```python
from build123d import *

# Parameters (mm, degrees)
SKETCH1_W           = 50
SKETCH1_H           = 40
BOSS_EXTRUDE1_DEPTH = 6
CUT_EXTRUDE3_DEPTH  = 4
SKETCH7_R           = 2
CUT_EXTRUDE4_DEPTH  = 6


with BuildPart() as part:
    # Sketch1 → Boss-Extrude1 (new body)
    with BuildSketch(Plane.XY):
        Rectangle(SKETCH1_W, SKETCH1_H)
    extrude(amount=BOSS_EXTRUDE1_DEPTH)

    # Sketch6 → Cut-Extrude3 (cut)
    with BuildSketch(Plane(origin=(0, 0, 0), x_dir=(-1, 0, 0), z_dir=(0, 0, -1))):
        with BuildLine():
            Line((-16.5, 15), (-16.5, -6))
            ThreePointArc((-16.5, -6), (-20, -9.5), (-23.5, -6))
            Line((-23.5, -6), (-23.5, 15))
            ThreePointArc((-23.5, 15), (-20, 18.5), (-16.5, 15))
        make_face()
        with BuildLine():
            Line((23.5, 15), (23.5, -6))
            ThreePointArc((23.5, -6), (20, -9.5), (16.5, -6))
            Line((16.5, -6), (16.5, 15))
            ThreePointArc((16.5, 15), (20, 18.5), (23.5, 15))
        make_face()
    extrude(amount=-CUT_EXTRUDE3_DEPTH, mode=Mode.SUBTRACT)

    # Sketch7 → Cut-Extrude4 (cut)
    with BuildSketch(Plane(origin=(0, 0, 0), x_dir=(-1, 0, 0), z_dir=(0, 0, -1))):
        with Locations((-20, -16.5)):
            Circle(SKETCH7_R)
        with Locations((20, -16.5)):
            Circle(SKETCH7_R)
        with BuildLine():
            Line((-22, 15), (-22, -6))
            ThreePointArc((-22, -6), (-20, -8), (-18, -6))
            Line((-18, -6), (-18, 15))
            ThreePointArc((-18, 15), (-20, 17), (-22, 15))
        make_face()
        with BuildLine():
            Line((18, 15), (18, -6))
            ThreePointArc((18, -6), (20, -8), (22, -6))
            Line((22, -6), (22, 15))
            ThreePointArc((22, 15), (20, 17), (18, 15))
        make_face()
    extrude(amount=-CUT_EXTRUDE4_DEPTH, mode=Mode.SUBTRACT)


solid = part.part
```
Part model, mm, in its own coordinate system. A direction names the side the tool comes from. Give positions to 0.01 mm unless a question says otherwise; leave off trailing zeros. Order: outer loops, then holes, each group sorted by start corner. A loop starts at its lowest first (then second) coordinate and runs counter-clockwise, first axis right, second up. Notation, with made-up numbers: M -6,-14 L 5,-14 A17 ccw 5,-6 Z; hole C -30,72.25 d6. An arc over 180 degrees is marked long. Use a Markdown table: item, result. Add a question column.
(1) Probe line 1 along Y through (x, z) = (20, 4.45); line 2 along X through (y, z) = (9, 0.6); line 3 along X through (y, z) = (10, 4.95). List the from-to ranges inside material, lowest first. Write a range as [from, to].
(2) Drop flat-ended pins along their axis: P1, Ø3, axis at x = -20, y = -16.5, coming from the -Z side; P2, Ø7.5, axis at x = -18.5, y = -2, coming from the -Z side. Give the stop position or say it passes through.
(3) Saw through at A-A, the plane x = 20. Give the cut face in (y, z).
(4) 3-axis set-ups, long thin cutter, end or side, ignore diameter. For faces 1 (the face through (0, 0, 0)), 2 (the face through (20, 17, 5)), 3 (the face through (16.5, 5, 2)): which of +Z, -Z, +X, -X, +Y, -Y reach the whole face in a straight line?
(5) Mould opens along Y. For faces 4 (the face through (-16.5, 4, 2)), 5 (the face through (0, 0, 6)), 6 (the face through (0, -20, 3)) say: +Y half, -Y half, draft (parallel to the pull), parting line (faces both ways), or undercut.
(6) Saw through at D-D, the plane z = 5.4. Give the cut face in (x, y), and give its area (3 significant figures).
(7) Saw through at C-C, the plane y = -3. Give the cut face in (x, z), and give its area (3 significant figures).
(8) Saw through at B-B, the plane z = 0.65. Give the cut face in (x, y), and give its area (3 significant figures).
Answer key:
| question | item | result |
|---|---|---|
| 1 | line 1 | [-20, -18.5], [-14.5, -8], [17, 20] |
| 1 | line 2 | [-25, -23.5], [-16.5, 16.5], [23.5, 25] |
| 1 | line 3 | [-25, -22], [-18, 18], [22, 25] |
| 2 | P1 | through |
| 2 | P2 | z = 0 |
| 3 | outline | M -20,0 L -18.5,0 L -18.5,6 L -20,6 Z; M -14.5,0 L -9.5,0 L -9.5,4 L -8,4 L -8,6 L -14.5,6 Z; M 17,4 L 18.5,4 L 18.5,0 L 20,0 L 20,6 L 17,6 Z |
| 4 | face 1 | -Z, +X, -X, +Y, -Y |
| 4 | face 2 | +Z, -Z |
| 4 | face 3 | -Z |
| 5 | face 4 | undercut |
| 5 | face 5 | draft |
| 5 | face 6 | -Y half |
| 6 | outline | M -25,-20 L 25,-20 L 25,20 L -25,20 Z; hole C -20,-16.5 d4; hole M -22,-6 A2 ccw -18,-6 L -18,15 A2 ccw -22,15 Z; hole C 20,-16.5 d4; hole M 18,-6 A2 ccw 22,-6 L 22,15 A2 ccw 18,15 Z |
| 6 | area | 1,780 mm^2 |
| 7 | outline | M -25,0 L -23.5,0 L -23.5,4 L -22,4 L -22,6 L -25,6 Z; M -18,4 L -16.5,4 L -16.5,0 L 16.5,0 L 16.5,4 L 18,4 L 18,6 L -18,6 Z; M 22,4 L 23.5,4 L 23.5,0 L 25,0 L 25,6 L 22,6 Z |
| 7 | area | 228 mm^2 |
| 8 | outline | M -25,-20 L 25,-20 L 25,20 L -25,20 Z; hole M -23.5,-6 A3.5 ccw -16.5,-6 L -16.5,15 A3.5 ccw -23.5,15 Z; hole C -20,-16.5 d4; hole M 16.5,-6 A3.5 ccw 23.5,-6 L 23.5,15 A3.5 ccw 16.5,15 Z; hole C 20,-16.5 d4 |
| 8 | area | 1,600 mm^2 |
